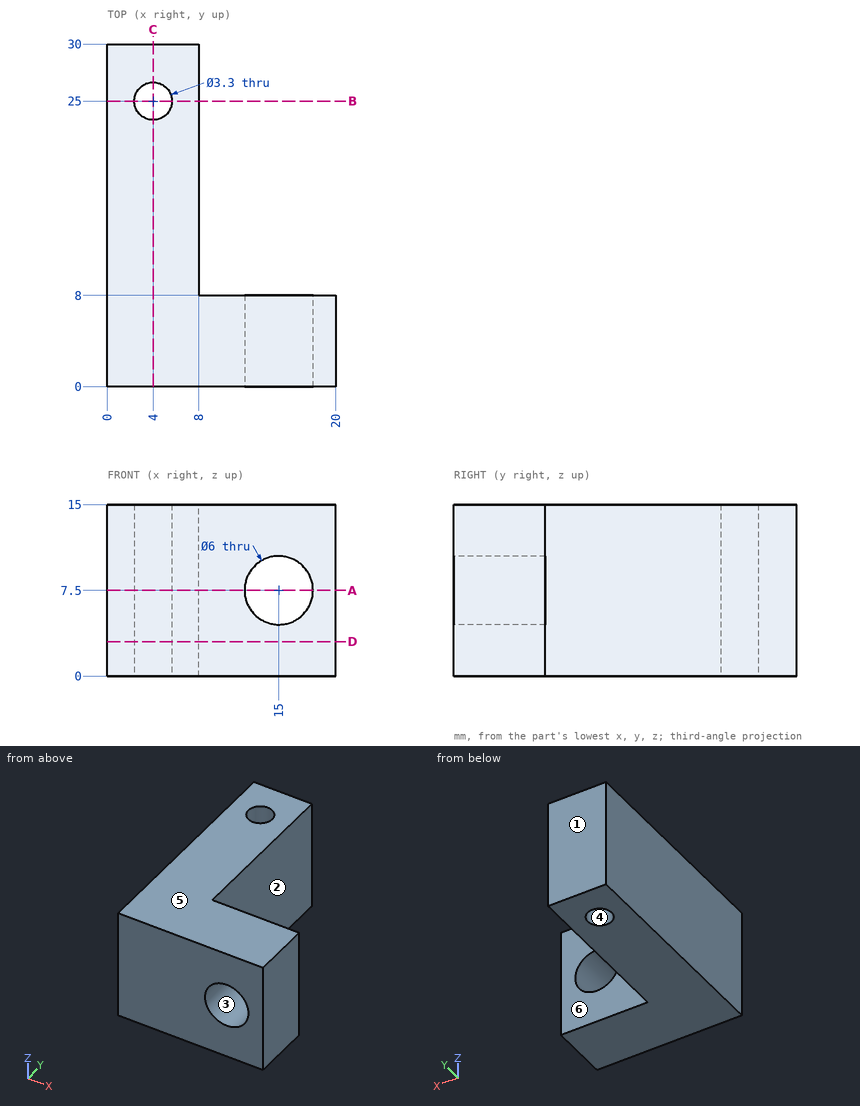
Here's the drawing with two shaded views (mm, measured from the low corner). I have some questions. A direction names the side the tool comes from. Round coordinates to 2 decimals unless told otherwise and drop trailing zeros. Order: outer loops, then holes, each group sorted by start corner. A loop starts at its lowest first (then second) coordinate and runs counter-clockwise, first axis right, second up. Notation, with made-up numbers: M 58.5,81.5 L 72.5,81.5 A9 cw 72.5,90.5 Z; hole C 85,68 d7. An arc over 180 degrees is marked long. Use CSV: the item, a comma, the result in double quotes.
1) I want a section at A-A (z = 7.5). List the corners of the cut face in (x, y) for me.
Taken from the geometry:
outline,"M 0,0 L 12,0 L 12,8 L 8,8 L 8,30 L 0,30 Z; M 18,0 L 20,0 L 20,8 L 18,8 Z; hole C 4,25 d3.3"
2) I'm going to push flat-ended pins straight in: P1, Ø5, axis at x = 16, z = 4.5, coming from the -Y side; P2, Ø2.5, axis at x = 4, y = 25, coming from the -Z side; P3, Ø7.5, axis at y = 22.5, z = 6, coming from the +X side. Where does each tip first touch, or does it pass through?
Taken from the geometry:
P1,"y = 0"
P2,"through"
P3,"x = 8"
3) I want a section at C-C (x = 4). List the corners of the cut face in (y, z) for me.
Taken from the geometry:
outline,"M 0,0 L 23.35,0 L 23.35,15 L 0,15 Z; M 26.65,0 L 30,0 L 30,15 L 26.65,15 Z"
4) I want a section at D-D (z = 3). List the corners of the cut face in (x, y) for me.
Taken from the geometry:
outline,"M 0,0 L 20,0 L 20,8 L 8,8 L 8,30 L 0,30 Z; hole C 4,25 d3.3"
5) On a 3-axis mill with a long thin cutter (end or side, diameter ignored), from which of +Z, -Z, +X, -X, +Y, -Y can I reach the whole of each face in a straight line? I mean the marked faces 5 and 6. Say none if no direction works.
Taken from the geometry:
face 5,"+Z, +X, -X, +Y, -Y"
face 6,"+Z, -Z, +X, +Y"
6) I need wall thicknesses on line 1 along Z through (x, y) = (15, 7.75); line 2 along Y through (x, z) = (17, 14.25); line 3 along Y through (x, z) = (4, 6.25). Which ranges of each line are inside material? Lowest first, please. Write a range as [from, to].
Taken from the geometry:
line 1,"[0, 4.5], [10.5, 15]"
line 2,"[0, 8]"
line 3,"[0, 23.35], [26.65, 30]"
7) If we mould it in two halves opening along X, with no side actions, what happens to the marked faces 1, 2, 3 and 4? For each: pulls with the +X half, pulls with the -X half, needs draft (parallel to the pull), parting line crosses it, or undercut.
Taken from the geometry:
face 1,"needs draft"
face 2,"pulls with the +X half"
face 3,"undercut"
face 4,"undercut"
8) I want a section at B-B (y = 25). List the corners of the cut face in (x, z) for me.
Taken from the geometry:
outline,"M 0,0 L 2.35,0 L 2.35,15 L 0,15 Z; M 5.65,0 L 8,0 L 8,15 L 5.65,15 Z"
